For this review, take the finished solid that the model builds, in its own axes (mm). A direction names the side the tool comes from. Round coordinates to 2 decimals unless told otherwise and drop trailing zeros. Order: outer loops, then holes, each group sorted by start corner. A loop starts at its lowest first (then second) coordinate and runs counter-clockwise, first axis right, second up. Notation, with made-up numbers: (20.5, 9) -> (78.5, 9) arc R21 ccw to (78.5, 42) -> close; hole circle Ø9 at (11.25, 2.5). An arc over 180 degrees is marked (long way). Use a Markdown table: item, result. Add a question column.
1) Wall thickness on line 1 along X through (y, z) = (-5, 32); line 2 along X through (y, z) = (-8, 9.5); line 3 along Y through (x, z) = (19, 34): over which ranges is each line inside the solid? List them lowest first. Write a range as [from, to].
2) Consider section C-C (x = -25.5). State the section outline as (y, z) points, plus the area to 3 significant figures.
3) Consider section A-A (y = -5). State the section outline as (x, z) points, plus the area to 3 significant figures.
4) Machinability: for faces 1 (the face through (0, 3, 18)), 2 (the face through (33, 0, 30)), 3 (the face through (-38, -3, 24)), 4 (the face through (0, 29, 10)), which of the approach directions +Z, -Z, +X, -X, +Y, -Y give a long, thin tool a straight path to every point of the face, cutting with its end or side? Answer none if there is none.
5) Consider section B-B (z = 7). State the section outline as (x, y) points.
6) Consider section D-D (y = 11). State the section outline as (x, z) points.
7) Draft analysis for pull direction X (two halves, no side actions). For faces 5 (the face through (15, -6, 18)), 6 (the face through (0, 8, 36)), 7 (the face through (-42, -7, 12)), state which applies: pulls with the +X half, pulls with the -X half, needs draft (parallel to the pull), parting line crosses it, or undercut.
8) Clearance check with flat-ended pins moving along their axes: P1, Ø8, axis at x = -1.5, z = 23, coming from the +Y side; P2, Ø10, axis at y = 23, z = 20, coming from the -X side; P3, Ø9.5, axis at y = -7.5, z = 28, coming from the -X side; P4, Ø2, axis at y = 8, z = 11, coming from the -X side. State where each tip first meets the part, or that it passes through.
```python
from build123d import *

# Parameters (mm, degrees)
SALIENTE_EXTRUIR1_DEPTH = 36
CORTAR_EXTRUIR1_DEPTH   = 26
CORTAR_EXTRUIR2_DEPTH   = 12
CROQUIS4_W              = 30
CROQUIS4_H              = 18
CORTAR_EXTRUIR3_DEPTH   = 66.459911396


with BuildPart() as part:
    # Croquis1 → Saliente-Extruir1 (new body)
    with BuildSketch(Plane.XY):
        Polygon((-42, -15), (42, -15), (42, 0), (20, 35), (-20, 35), (-42, 0), align=None)
    extrude(amount=SALIENTE_EXTRUIR1_DEPTH)

    # Croquis2 → Cortar-Extruir1 (cut)
    with BuildSketch(Plane.XY.offset(36)):
        Polygon((-20, 35), (-27.542857143, 23), (27.542857143, 23), (20, 35), align=None)
    extrude(amount=-CORTAR_EXTRUIR1_DEPTH, mode=Mode.SUBTRACT)

    # Croquis3 → Cortar-Extruir2 (cut)
    with BuildSketch(Plane.XY.offset(36)):
        Polygon((33, 14.318181818), (33, -15), (42, -15), (42, 0), align=None)
        Polygon((-33, -15), (-33, 14.318181818), (-42, 0), (-42, -15), align=None)
    extrude(amount=-CORTAR_EXTRUIR2_DEPTH, mode=Mode.SUBTRACT)

    # Croquis4 → Cortar-Extruir3 (cut, through all)
    with BuildSketch(Plane.XY.offset(36)):
        with Locations((0, -6)):
            Rectangle(CROQUIS4_W, CROQUIS4_H)
    extrude(amount=-CORTAR_EXTRUIR3_DEPTH, mode=Mode.SUBTRACT)


solid = part.part
```
Results list:
| question | item | result |
|---|---|---|
| 1 | line 1 | [-33, -15], [15, 33] |
| 1 | line 2 | [-42, -15], [15, 42] |
| 1 | line 3 | [-15, 23] |
| 2 | outline | (-15, 0) -> (26.25, 0) -> (26.25, 10) -> (23, 10) -> (23, 36) -> (-15, 36) -> close |
| 2 | area | 1,400 mm2 |
| 3 | outline | (-42, 0) -> (-15, 0) -> (-15, 36) -> (-33, 36) -> (-33, 24) -> (-42, 24) -> close; (15, 0) -> (42, 0) -> (42, 24) -> (33, 24) -> (33, 36) -> (15, 36) -> close |
| 3 | area | 1,730 mm2 |
| 4 | face 1 | +Z, -Z, -Y |
| 4 | face 2 | +Z, +X, +Y, -Y |
| 4 | face 3 | +Z, -X, +Y, -Y |
| 4 | face 4 | +Z, +X, -X, +Y |
| 5 | outline | (-42, -15) -> (-15, -15) -> (-15, 3) -> (15, 3) -> (15, -15) -> (42, -15) -> (42, 0) -> (20, 35) -> (-20, 35) -> (-42, 0) -> close |
| 6 | outline | (-35.09, 0) -> (35.09, 0) -> (35.09, 24) -> (33, 24) -> (33, 36) -> (-33, 36) -> (-33, 24) -> (-35.09, 24) -> close |
| 7 | face 5 | undercut |
| 7 | face 6 | needs draft |
| 7 | face 7 | pulls with the -X half |
| 8 | P1 | y = 23 |
| 8 | P2 | x = -30.69 |
| 8 | P3 | x = -42 |
| 8 | P4 | x = -37.6 |
